from build123d import *

# Parameters (mm, degrees)
SKETCH1_W           = 10
SKETCH1_H           = 70
BOSS_EXTRUDE1_DEPTH = 3
BOSS_EXTRUDE2_DEPTH = 3
SKETCH3_R           = 5
SKETCH3_R_2         = 1.25
CUT_EXTRUDE1_DEPTH  = 4


with BuildPart() as part:
    # Sketch1 → Boss-Extrude1 (new body)
    with BuildSketch(Plane.XY):
        with Locations((-30.31593178, 0.053868552)):
            Rectangle(SKETCH1_W, SKETCH1_H)
    extrude(amount=BOSS_EXTRUDE1_DEPTH)

    # Sketch2 → Boss-Extrude2 (add)
    with BuildSketch(Plane.XY.offset(3)):
        Polygon((-40.31593178, -39.946131448), (-40.31593178, -27.079464781), (-50.31593178, -11.346131448), (-50.31593178, 3.653868552), (-42.81593178, 35.053868552), (-35.31593178, 35.053868552), (-35.31593178, -34.946131448), (-35.31593178, -39.946131448), align=None)
    extrude(amount=-BOSS_EXTRUDE2_DEPTH)

    # Sketch3 → Cut-Extrude1 (cut, through all)
    with BuildSketch(Plane.XY.offset(3)):
        with Locations((-42.81593178, -3.846131448)):
            Circle(SKETCH3_R)
        with Locations((-32.31593178, -30.946131448)):
            Circle(SKETCH3_R_2)
        Polygon((-35.31593178, -34.946131448), (-25.31593178, -33.182379001), (-25.31593178, -34.946131448), align=None)
    extrude(amount=-CUT_EXTRUDE1_DEPTH, mode=Mode.SUBTRACT)


solid = part.part
Work out the finished part from the listing and answer in its coordinate system (mm). A direction names the side the tool comes from. Round coordinates to 2 decimals unless told otherwise and drop trailing zeros. Write each loop counter-clockwise with the first axis right and the second up, starting at its lowest first coordinate (ties: lowest second). Pieces come first, ordered by that corner, then holes. Notation, with made-up numbers: (-11, -15) -> (42, -15) arc R9 cw to (42, -9) -> close; hole circle Ø1 at (64, 35.25). An arc over 180 degrees is marked (long way). Answer as CSV lines item,"result". Start each with the question number.
(1) The part is cut by section A-A, the plane x = -38.75. Give the vertices of the cut face in (y, z), then the cut area to 3 significant figures.
(2) Find the intervals of material crossed by probe 1 along X at (y, z) = (-28.5, 1.7); probe 2 along Y at (x, z) = (-33, 2.8); probe 3 along Y at (x, z) = (-41.5, 2.65), in increasing order.
(3) The part is cut by section D-D, the plane x = -32.75. Give the vertices of the cut face in (y, z), then the cut area to 3 significant figures.
(4) Each of these flat-tipped pins is pushed along its axis until it touches: pin 1 (1.5 mm diameter, centred on y = -37.5, z = 2, fed in from +X); pin 2 (1.5 mm diameter, centred on y = -33.5, z = 1, fed in from -X); pin 3 (6 mm diameter, centred on x = -45, y = -19, fed in from -Z). Where does it stop, or does it pass through?
(5) The part is cut by section B-B, the plane z = 1.75. Give the vertices of the cut face in (x, y), then the cut area to 3 significant figures.
(6) The mould has two halves that part along Y. Classify faces 3 (the flat face through (-40.316, -34, 2)), 4 (the cylindrical face through (-33.308, -31.707, 1.521)), 5 (the flat face through (-30.386, -34.077, 1.521)): +Y half, -Y half, draft (parallel to the pull), parting line (faces both ways), or undercut.
(7) A tool of negligible diameter and unlimited length cuts with its end or side. For faces 1 (the flat face through (-35.316, -37, 2)), 2 (the flat face through (-50.316, -4, 2)), from which of +Z, -Z, +X, -X, +Y, -Y can it reach the whole face along a straight path? Write none if from no direction.
(8) The part is cut by section C-C, the plane y = -29. Give the vertices of the cut face in (x, z).
Output values:
1,outline,"(-39.95, 0) -> (-6.76, 0) -> (-6.76, 3) -> (-39.95, 3) -> close; (-0.94, 0) -> (35.05, 0) -> (35.05, 3) -> (-0.94, 3) -> close"
1,area,"208 mm²"
2,probe 1,"x = -40.32 to -25.32"
2,probe 2,"y = -34.54 to -31.99, -29.9 to 35.05"
2,probe 3,"y = -25.22 to -8.67, 0.98 to 35.05"
3,outline,"(-34.49, 0) -> (-32.12, 0) -> (-32.12, 3) -> (-34.49, 3) -> close; (-29.77, 0) -> (35.05, 0) -> (35.05, 3) -> (-29.77, 3) -> close"
3,area,"202 mm²"
4,pin 1,"stops at x = -35.32"
4,pin 2,"stops at x = -40.32"
4,pin 3,"stops at z = 0"
5,outline,"(-50.32, -11.35) -> (-40.32, -27.08) -> (-40.32, -39.95) -> (-35.32, -39.95) -> (-35.32, -34.95) -> (-25.32, -33.18) -> (-25.32, 35.05) -> (-42.82, 35.05) -> (-50.32, 3.65) -> close; hole circle Ø10 at (-42.82, -3.85); hole circle Ø2.5 at (-32.32, -30.95)"
5,area,"1,410 mm²"
6,face 3,"draft"
6,face 4,"undercut"
6,face 5,"-Y half"
7,face 1,"+Z, -Z, +X, -Y"
7,face 2,"+Z, -Z, -X, +Y, -Y"
8,outline,"(-40.32, 0) -> (-25.32, 0) -> (-25.32, 3) -> (-40.32, 3) -> close"
